Part print with two shaded views. Sizes in mm from the minimum x, y, z corner. A direction names the side the tool comes from. Give positions to 0.01 mm unless a question says otherwise; leave off trailing zeros. Loops run counter-clockwise (first coordinate to the right, second up) from the corner with the lowest first, then second, coordinate; pieces in that order, holes last. Notation, with made-up numbers: (-33, 73.5) -> (-13, 73.5) arc R13 ccw to (-13, 95.5) -> close; hole circle Ø5 at (-32.75, 35). An arc over 180 degrees is marked (long way). One line per question, with ' | ' between items.
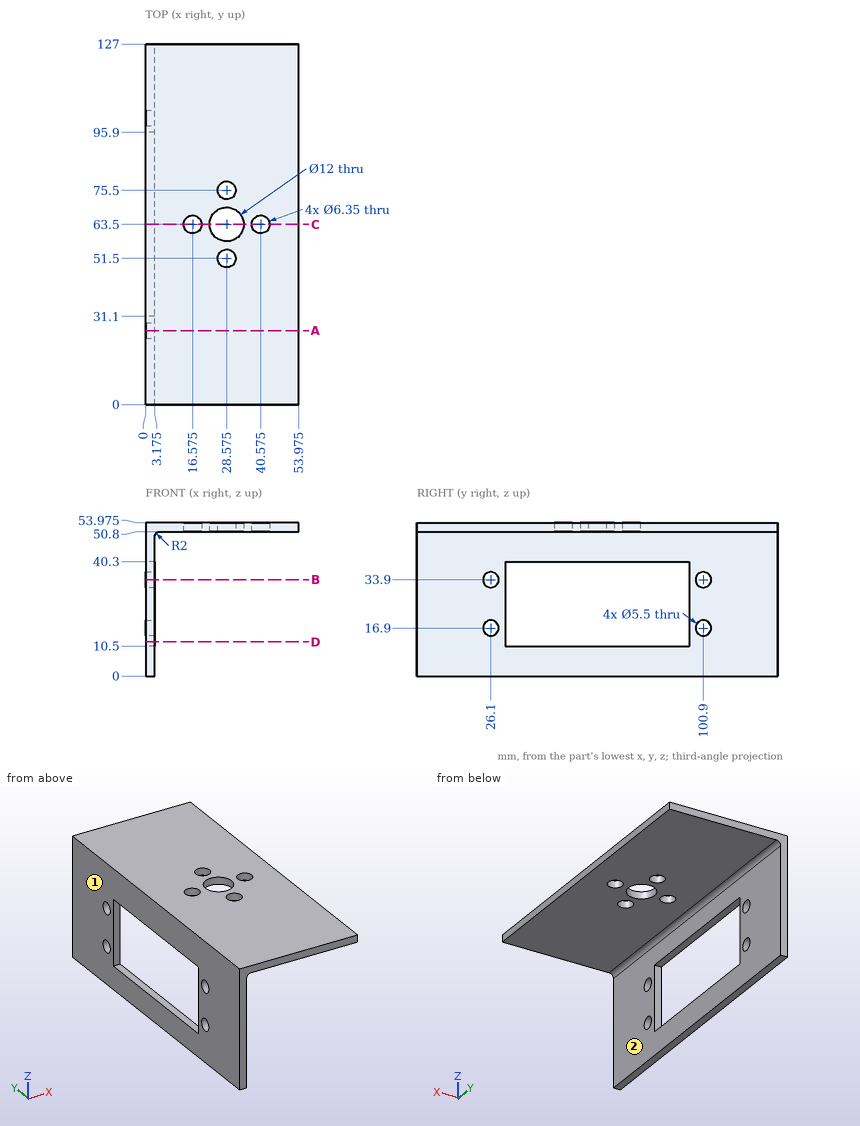
1) Pin check, flat tips, straight feed: P1, Ø1.6, axis at x = 1.5, y = 56.5, coming from the -Z side; P2, Ø7, axis at y = 26.1, z = 16.9, coming from the +X side (3 decimals); P3, Ø14.5, axis at x = 36.5, y = 52, coming from the -Z side. Stop position of each tip, or through.
Found:
P1: z = 0 | P2: x = 3.175 | P3: z = 50.8
2) Tool access for the marked faces 1 and 2: list every direction of +Z, -Z, +X, -X, +Y, -Y with a clear straight run to the whole face (end or side of a thin tool).
Found:
face 1: +Z, -Z, -X, +Y, -Y | face 2: -Z, +X, +Y, -Y
3) Saw through at D-D (z = 12). Give the cut face in (x, y) (3 decimals), and give its area (3 significant figures).
Found:
outline: (0, 0) -> (3.175, 0) -> (3.175, 31.1) -> (0, 31.1) -> close; (0, 95.9) -> (3.175, 95.9) -> (3.175, 127) -> (0, 127) -> close | area: 197 mm2
4) Drill centre lines: line 1 (Y direction, x = 1.8, z = 33.9); line 2 (Z direction, x = 31.5, y = 108) (3 decimals); line 3 (X direction, y = 119, z = 30) (3 decimals). Where is each one in solid material? Low to high.
Found:
line 1: 0 to 23.35, 28.85 to 31.1, 95.9 to 98.15, 103.65 to 127 | line 2: 50.8 to 53.975 | line 3: 0 to 3.175
5) Saw through at C-C (y = 63.5). Give the cut face in (x, z) (3 decimals), and give its area (3 significant figures).
Found:
outline: (0, 0) -> (3.175, 0) -> (3.175, 10.5) -> (0, 10.5) -> close; (0, 40.3) -> (3.175, 40.3) -> (3.175, 48.8) arc R2 cw to (5.175, 50.8) -> (13.4, 50.8) -> (13.4, 53.975) -> (0, 53.975) -> close; (19.75, 50.8) -> (22.575, 50.8) -> (22.575, 53.975) -> (19.75, 53.975) -> close; (34.575, 50.8) -> (37.4, 50.8) -> (37.4, 53.975) -> (34.575, 53.975) -> close; (43.75, 50.8) -> (53.975, 50.8) -> (53.975, 53.975) -> (43.75, 53.975) -> close | area: 160 mm2
6) Saw through at B-B (z = 33.9). Give the cut face in (x, y) (3 decimals), and give its area (3 significant figures).
Found:
outline: (0, 0) -> (3.175, 0) -> (3.175, 23.35) -> (0, 23.35) -> close; (0, 28.85) -> (3.175, 28.85) -> (3.175, 31.1) -> (0, 31.1) -> close; (0, 95.9) -> (3.175, 95.9) -> (3.175, 98.15) -> (0, 98.15) -> close; (0, 103.65) -> (3.175, 103.65) -> (3.175, 127) -> (0, 127) -> close | area: 163 mm2
7) Saw through at A-A (y = 26.1). Give the cut face in (x, z) (3 decimals), and give its area (3 significant figures).
Found:
outline: (0, 0) -> (3.175, 0) -> (3.175, 14.15) -> (0, 14.15) -> close; (0, 19.65) -> (3.175, 19.65) -> (3.175, 31.15) -> (0, 31.15) -> close; (0, 36.65) -> (3.175, 36.65) -> (3.175, 48.8) arc R2 cw to (5.175, 50.8) -> (53.975, 50.8) -> (53.975, 53.975) -> (0, 53.975) -> close | area: 299 mm2
